Autodesk Inventor part; units mm, degrees
ref_plane "YZ Plane" through (0, 0, 0) normal (1, 0, 0) x (0, 1, 0)
ref_plane "XZ Plane" through (0, 0, 0) normal (0, 1, 0) x (-1, 0, 0)
ref_plane "XY Plane" through (0, 0, 0) normal (0, 0, 1) x (1, 0, 0)
sketch "Sketch1" plane through (0, 0, 0) normal (0, 1, 0) x (-1, 0, 0)
  line L0 (0, 0) -> (0, -16)
  line L1 (0, 0) -> (0, -30)
  line L2 (0, -16) -> (0, -20)
  line L3 (0, -16) -> (50, -16)
  line L4 (50, -16) -> (50, 0)
  line L5 (50, 0) -> (0, 0)
  line L6 (50, -20) -> (50, -16)
  arc A0 (0.5833, -23.0243) -> (0.5833, -36.9757) centre (0, -30) ccw
  line L7 (0, -30) -> (30, -30)
  circle A1 centre (30, -30) radius 4.5
  line L8 (30.375, -25.5157) -> (0.5833, -23.0243)
  line L9 (30.375, -34.4843) -> (0.5833, -36.9757)
  line L10 (0, -40) -> (45, -40)
  line L11 (45, -40) -> (45, -20)
  line L12 (45, -20) -> (0, -20)
  circle A2 centre (30, -30) radius 1.7
  circle A3 centre (15, -30) radius 1.7
  line L13 (45, -30) -> (40, -30)
  circle A4 centre (40, -30) radius 1.7
  circle A5 centre (0, -30) radius 3.15
  circle A6 centre (0, -30) radius 1.7
  line L14 (45, -20) -> (0, -20)
  line L15 (45, -20) -> (35.5, -20)
  line L16 (35.5, -20) -> (35.5, -40)
  arc A7 (0, -20) -> (0, -40) centre (0, -30) ccw
  dimension "d0" = 16
  dimension "d1" = 30
  dimension "d2" = 4
  dimension "d3" = 50
  dimension "d4" = 50
  dimension "d22" = 14
  dimension "d23" = 30
  dimension "d24" = 9
  dimension "d26" = 45
  dimension "d29" = 3.4
  dimension "d30" = 3.4
  dimension "d31" = 5
  dimension "d32" = 3.4
  dimension "d34" = 6.3
  dimension "d35" = 3.4
  dimension "d36" = 9.5
extrude "Extrusion4" add sketch "Sketch1" along normal blind 16 contours A0 L8 A1 L7 A3 A5 L1 | L1 A5 L7 A3 A1 L9 A0 | A5 L7 A6 L1 | L1 A6 L7 A5 | A1
extrude "Extrusion5" add sketch "Sketch1" along normal blind 19 contours L12 L16 L10 A7
extrude "Extrusion6" add sketch "Sketch1" along normal blind 12 contours L12 L11 L10 L16
extrude "Extrusion7" cut sketch "Sketch1" along normal blind 5 contours A5 L7 A6 L1 | L1 A6 L7 A5
properties part number "servo_clip1"
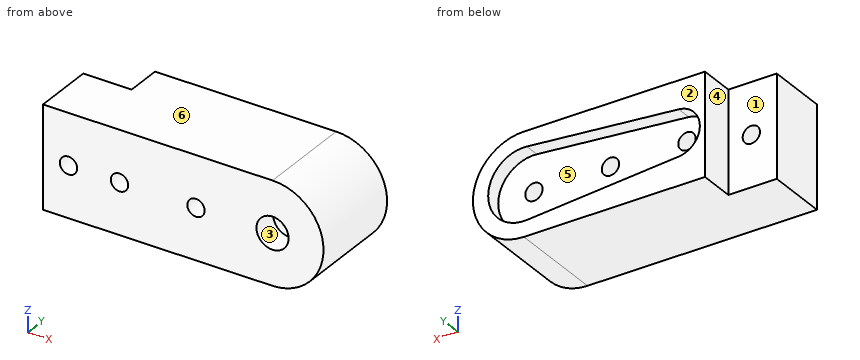
The model under review builds one solid part; all positions refer to its coordinate system, in mm. Face numbers are marked on the shaded views. A direction names the side the tool comes from. Give positions to 0.01 mm unless a question says otherwise; leave off trailing zeros. Order: outer loops, then holes, each group sorted by start corner. A loop starts at its lowest first (then second) coordinate and runs counter-clockwise, first axis right, second up. Notation, with made-up numbers: M -30,38.25 L 16,38.25 A17 ccw 16,52.25 Z; hole C 22,81.5 d10. An arc over 180 degrees is marked long. Use one line per item in the form item = value. Start each with the question number.
Item 1: We need section D-D on y = 17.5. Give the boundary of the cut face in (x, z) (3 decimals), plus the area to 3 significant figures.
Item 2: The part is to be moulded in two halves that separate along Z. For the marked faces 4, 5 and 6, say which applies: pulls with the +Z half, pulls with the -Z half, needs draft (parallel to the pull), parting line crosses it, or undercut.
Item 3: Insertion check: pin 1 Ø10 at (x, z) = (-9, -36) entering from +Y; pin 2 Ø1.5 at (x, z) = (-30, -30.5) entering from +Y; pin 3 Ø3 at (x, z) = (2, -30) entering from +Y; pin 4 Ø3 at (x, z) = (-38, -25.5) entering from +Y. Each pin has a flat end and moves straight along its axis. Give the tip position at first contact, or say it passes through.
Item 4: To check wall thickness, follow line 1 along Z through (x, y) = (-40, 9.5); line 2 along X through (y, z) = (13.75, -29); line 3 along Z through (x, y) = (0, 17.05). State the ranges of each line that lie inside material, in increasing order. Write a range as from..to.
Item 5: We need section A-A on x = -40. Give the boundary of the cut face in (y, z), plus the area to 3 significant figures.
Item 6: We need section C-C on z = -30. Give the number of separate pieces and of enclosed holes in the cut face, plus the area to 4 significant figures.
Item 7: For the marked faces 1, 2 and 3, list the 3-axis set-ups (+Z, -Z, +X, -X, +Y, -Y) from which the entire face can be reached by the end or side of a thin tool; tool diameter is ignored.
Item 8: We need section B-B on y = 10. Give the boundary of the cut face in (x, z).
Completed:
q1.outline = M -35.5,-40 L 0,-40 A10 ccw 0,-20 L -35.5,-20 Z; hole M -30.375,-34.484 L -0.583,-36.976 A7 ccw long -0.583,-23.024 L -30.375,-25.516 A4.5 ccw Z
q1.area = 412 mm²
q2.face_4 = needs draft
q2.face_5 = undercut
q2.face_6 = pulls with the +Z half
q3.pin_1 = 19
q3.pin_2 = through
q3.pin_3 = 16
q3.pin_4 = 12
q4.line_1 = -40..-31.7, -28.3..-20
q4.line_2 = -35.5..-31.37, -28.63..-16.37, -13.63..-1.37, 1.37..9.95
q4.line_3 = -40..-37, -23..-20
q5.outline = M 0,-40 L 12,-40 L 12,-31.7 L 0,-31.7 Z; M 0,-28.3 L 12,-28.3 L 12,-20 L 0,-20 Z
q5.area = 199 mm²
q6.separate_pieces = 5
q6.enclosed_holes = 0
q6.area = 635.5 mm²
q7.face_1 = +Z, -Z, -X, +Y
q7.face_2 = +Z, -Z, +X, -X, +Y
q7.face_3 = -Y
q8.outline = M -45,-40 L 0,-40 A10 ccw 0,-20 L -45,-20 Z; hole C -40,-30 d3.4; hole C -30,-30 d3.4; hole C -15,-30 d3.4; hole C 0,-30 d3.4
